The listing builds one solid part. Answer for the finished solid, in the listing's coordinates (mm). Coordinates: 2 decimals unless noted, no trailing zeros. Order: outer loops, then holes, each group sorted by start corner. A loop starts at its lowest first (then second) coordinate and runs counter-clockwise, first axis right, second up. Notation, with made-up numbers: (61, -36.75) - (94, -36.75) arc R18 cw to (94, -29.75) - close; hole circle Ø9 at (38, 37). An arc over 180 degrees is marked (long way). Use a Markdown table: item, result. Add a question column.
Item 1: The part is cut by section C-C, the plane y = 2.5. Give the vertices of the cut face in (x, z).
Item 2: The part is cut by section B-B, the plane z = 1. Give the vertices of the cut face in (x, y).
Item 3: The mould has two halves that part along Y. Classify faces 1 (the flat face through (24, 0, 0)), 2 (the cylindrical face through (-3, 0, 3)), 3 (the cylindrical face through (45, 0, 3)), 4 (the flat face through (24, -5, 3)): released by +Y, released by -Y, zero draft, split by the parting line, or undercut.
Item 4: Flat-ended cylindrical pins translate along their axes: P1, Ø2, axis at y = 0.5, z = 1, coming from the +X side; P2, Ø1, axis at y = 3, z = 2, coming from the -X side; P3, Ø1, axis at y = 2, z = 1, coming from the +X side. Find the tip coordinate at first contact, or state that the pin passes through.
Item 5: The part is cut by section D-D, the plane y = -4.5. Give the vertices of the cut face in (x, z), then the cut area to 3 significant figures.
Item 6: The part is cut by section A-A, the plane y = 0. Give the vertices of the cut face in (x, z), then the cut area to 3 significant figures.
Item 7: Find the intervals of material crossed by line 1 along Y through (x, z) = (0, 1.6); line 2 along Y through (x, z) = (47, 4.5); line 3 along X through (y, z) = (-3.75, 3.8), in increasing order.
from build123d import *

# Parameters (mm, degrees)
SKETCH1_R           = 3
BOSS_EXTRUDE1_DEPTH = 6


with BuildPart() as part:
    # Sketch1 → Boss-Extrude1 (new body)
    with BuildSketch(Plane.XY):
        with BuildLine():
            ThreePointArc((0, 5), (-5, 0), (0, -5))
            Line((0, -5), (48, -5))
            ThreePointArc((48, -5), (53, 0), (48, 5))
            Line((48, 5), (0, 5))
        make_face()
        Circle(SKETCH1_R, mode=Mode.SUBTRACT)
        with Locations((48, 0)):
            Circle(SKETCH1_R, mode=Mode.SUBTRACT)
    extrude(amount=BOSS_EXTRUDE1_DEPTH)


solid = part.part
Solution:
| question | item | result |
|---|---|---|
| 1 | outline | (-4.33, 0) - (-1.66, 0) - (-1.66, 6) - (-4.33, 6) - close; (1.66, 0) - (46.34, 0) - (46.34, 6) - (1.66, 6) - close; (49.66, 0) - (52.33, 0) - (52.33, 6) - (49.66, 6) - close |
| 2 | outline | (0, -5) - (48, -5) arc R5 ccw to (48, 5) - (0, 5) arc R5 ccw to start; hole circle Ø6 at (0, 0); hole circle Ø6 at (48, 0) |
| 3 | face 1 | zero draft |
| 3 | face 2 | undercut |
| 3 | face 3 | undercut |
| 3 | face 4 | released by -Y |
| 4 | P1 | stops at x = 53 |
| 4 | P2 | stops at x = -4.33 |
| 4 | P3 | stops at x = 52.77 |
| 5 | outline | (-2.18, 0) - (50.18, 0) - (50.18, 6) - (-2.18, 6) - close |
| 5 | area | 314 mm2 |
| 6 | outline | (-5, 0) - (-3, 0) - (-3, 6) - (-5, 6) - close; (3, 0) - (45, 0) - (45, 6) - (3, 6) - close; (51, 0) - (53, 0) - (53, 6) - (51, 6) - close |
| 6 | area | 276 mm2 |
| 7 | line 1 | y = -5 to -3, 3 to 5 |
| 7 | line 2 | y = -5 to -2.83, 2.83 to 5 |
| 7 | line 3 | x = -3.31 to 51.31 |
